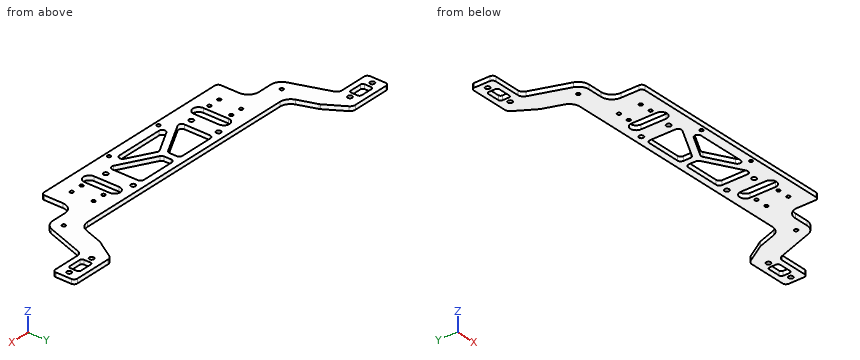
```python
from build123d import *

# Parameters (mm, degrees)
SKETCH_1_W           = 196
SKETCH_1_H           = 49.67
EXTRUDE_1_DEPTH      = 4
EXTRUDE_2_DEPTH      = 4
FILLET_1_R           = 10
FILLET_2_R           = 3
SKETCH_4_R           = 2.1
CUT_EXTRUDE_2_DEPTH  = 4
FILLET_3_R           = 5
SKETCH_5_R           = 1.55
CUT_EXTRUDE_3_DEPTH  = 10
SKETCH_7_R           = 2.05
CUT_EXTRUDE_5_DEPTH  = 102
CUT_EXTRUDE_8_DEPTH  = 10
FILLET_4_R           = 3
SKETCH_15_W          = 6
SKETCH_15_H          = 20
EXTRUDE_4_DEPTH      = 4
FILLET_11_R          = 10
FILLET_12_R          = 2
SKETCH_16_R          = 1.6
CUT_EXTRUDE_13_DEPTH = 10
SKETCH_23_W          = 16
SKETCH_23_H          = 22
CUT_EXTRUDE_17_DEPTH = 10
SKETCH_24_R          = 1.6
EXTRUDE_6_DEPTH      = 4
FILLET_14_R          = 10
SKETCH_25_W          = 15
SKETCH_25_H          = 10
CUT_EXTRUDE_18_DEPTH = 10
SKETCH_27_R          = 1.55
CUT_EXTRUDE_19_DEPTH = 5
SKETCH_30_R          = 1.6
CUT_EXTRUDE_22_DEPTH = 10
FILLET_15_R          = 2
CUT_EXTRUDE_23_DEPTH = 10


with BuildPart() as part:
    # 草图1 → 凸台-拉伸1 (new body)
    with BuildSketch(Plane.XY):
        Rectangle(SKETCH_1_W, SKETCH_1_H)
    extrude(amount=EXTRUDE_1_DEPTH)

    # 草图2 → 凸台-拉伸2 (add)
    with BuildSketch(Plane.XY.offset(4)):
        Polygon((98, 24.835), (114, 24.835), (122.222543405, 48.715), (134.566612912, 68.715), (174.566612912, 68.715), (174.566612912, 48.715), (143.374957029, 48.715), (128.265861358, 4.835), (98, 4.835), align=None)
        Polygon((-98, 24.835), (-98, 4.835), (-128.265861358, 4.835), (-143.374957029, 48.715), (-174.566612912, 48.715), (-174.566612912, 68.715), (-134.566612912, 68.715), (-122.222543405, 48.715), (-114, 24.835), align=None)
    extrude(amount=-EXTRUDE_2_DEPTH)

    # 圆角1
    fillet_1_edges = [part.edges().sort_by_distance(p)[0] for p in [
        (128.265861358, 4.835, 2),
        (114, 24.835, 2),
        (-128.265861358, 4.835, 2),
        (-114, 24.835, 2),
    ]]
    fillet(fillet_1_edges, radius=FILLET_1_R)

    # 圆角2
    fillet_2_edges = [part.edges().sort_by_distance(p)[0] for p in [
        (174.566612912, 48.715, 2),
        (174.566612912, 68.715, 2),
        (-174.566612912, 68.715, 2),
        (-174.566612912, 48.715, 2),
        (98, -24.835, 2),
        (-98, -24.835, 2),
    ]]
    fillet(fillet_2_edges, radius=FILLET_2_R)

    # 草图4 → 切除-拉伸2 (cut)
    with BuildSketch(Plane.XY.offset(4)):
        with Locations((47.5, -7.338706147)):
            Circle(SKETCH_4_R)
        with Locations((47.5, 17.661293853)):
            Circle(SKETCH_4_R)
        with Locations((-47.5, 17.661293853)):
            Circle(SKETCH_4_R)
        with Locations((-47.5, -7.338706147)):
            Circle(SKETCH_4_R)
    extrude(amount=-CUT_EXTRUDE_2_DEPTH, mode=Mode.SUBTRACT)

    # 圆角3
    fillet_3_edges = [part.edges().sort_by_distance(p)[0] for p in [
        (143.374957029, 48.715, 2),
        (134.566612912, 68.715, 2),
        (122.222543405, 48.715, 2),
        (-122.222543405, 48.715, 2),
        (-134.566612912, 68.715, 2),
        (-143.374957029, 48.715, 2),
    ]]
    fillet(fillet_3_edges, radius=FILLET_3_R)

    # 草图5 → 切除-拉伸3 (cut)
    with BuildSketch(Plane.XY.offset(4)):
        with Locations((27.5, -20.895)):
            Circle(SKETCH_5_R)
        with Locations(Location((-27.5, -20.895, 0), (0, 0, 180))):
            Circle(SKETCH_5_R)
    extrude(amount=-CUT_EXTRUDE_3_DEPTH, mode=Mode.SUBTRACT)

    # 草图7 → 切除-拉伸5 (cut)
    with BuildSketch(Plane.XY.offset(4)):
        with Locations((-168.566612912, 58.715)):
            Circle(SKETCH_7_R)
        with Locations((-143.566612912, 58.715)):
            Circle(SKETCH_7_R)
        with Locations(Location((143.566612912, 58.715, 0), (0, 0, 180))):
            Circle(SKETCH_7_R)
        with Locations(Location((168.566612912, 58.715, 0), (0, 0, 180))):
            Circle(SKETCH_7_R)
    extrude(amount=-CUT_EXTRUDE_5_DEPTH, mode=Mode.SUBTRACT)

    # 草图8 → 切除-拉伸8 (cut)
    with BuildSketch(Plane.XY.offset(4)):
        Polygon((-40, 18.835), (-40, -12.480899084), (-3, 7.619350916), (-3, 18.835), align=None)
        Polygon((0, 2.420899084), (-33.715414789, -15.895), (33.715414789, -15.895), align=None)
        Polygon((3, 7.619350916), (40, -12.480899084), (40, 18.835), (3, 18.835), align=None)
    extrude(amount=-CUT_EXTRUDE_8_DEPTH, mode=Mode.SUBTRACT)

    # 圆角4
    fillet_4_edges = [part.edges().sort_by_distance(p)[0] for p in [
        (0, 2.420899084, 2),
        (33.715414789, -15.895, 2),
        (-33.715414789, -15.895, 2),
        (3, 7.619350916, 2),
        (3, 18.835, 2),
        (40, 18.835, 2),
        (40, -12.480899084, 2),
        (-3, 7.619350916, 2),
        (-40, -12.480899084, 2),
        (-40, 18.835, 2),
        (-3, 18.835, 2),
    ]]
    fillet(fillet_4_edges, radius=FILLET_4_R)

    # 草图15 → 凸台-拉伸4 (add)
    with BuildSketch(Plane(origin=(0, 0, 0), x_dir=(-1, 0, 0), z_dir=(0, 0, -1))):
        with Locations((-101, -5.165)):
            Rectangle(SKETCH_15_W, SKETCH_15_H)
    extrude_4 = extrude(amount=-EXTRUDE_4_DEPTH)

    # 镜向5: 凸台-拉伸4 across plane
    add(extrude_4.mirror(Plane(origin=(0, 0, 0), x_dir=(0, 0, 1), z_dir=(1, 0, 0))))

    # 圆角11
    fillet_11_edges = [part.edges().sort_by_distance(p)[0] for p in [
        (104, 4.835, 2),
        (-104, 4.835, 2),
    ]]
    fillet(fillet_11_edges, radius=FILLET_11_R)

    # 圆角12
    fillet_12_edges = [part.edges().sort_by_distance(p)[0] for p in [
        (98, -15.165, 2),
        (104, -15.165, 2),
        (-104, -15.165, 2),
        (-98, -15.165, 2),
    ]]
    fillet(fillet_12_edges, radius=FILLET_12_R)

    # 草图16 → 切除-拉伸13 (cut)
    with BuildSketch(Plane.XY.offset(4)):
        with Locations((104, -10.165)):
            Circle(SKETCH_16_R)
        with Locations((104, 9.835)):
            Circle(SKETCH_16_R)
    cut_extrude_13 = extrude(amount=-CUT_EXTRUDE_13_DEPTH, mode=Mode.SUBTRACT)

    # 镜向6: 切除-拉伸13 across plane
    add(cut_extrude_13.mirror(Plane(origin=(0, 0, 0), x_dir=(0, 0, 1), z_dir=(1, 0, 0))), mode=Mode.SUBTRACT)

    # 草图23 → 切除-拉伸17 (cut)
    with BuildSketch(Plane.XY.offset(4)):
        with Locations((-106, -6.165)):
            Rectangle(SKETCH_23_W, SKETCH_23_H)
        with Locations((106, -6.165)):
            Rectangle(SKETCH_23_W, SKETCH_23_H)
    extrude(amount=-CUT_EXTRUDE_17_DEPTH, mode=Mode.SUBTRACT)

    # 草图24 → 凸台-拉伸6 (add)
    with BuildSketch(Plane.XY.offset(4)):
        with Locations((104, 9.835)):
            Circle(SKETCH_24_R)
        with Locations((-104, 9.835)):
            Circle(SKETCH_24_R)
    extrude(amount=-EXTRUDE_6_DEPTH)

    # 圆角14
    fillet_14_edges = [part.edges().sort_by_distance(p)[0] for p in [
        (-98, 4.835, 2),
        (98, 4.835, 2),
    ]]
    fillet(fillet_14_edges, radius=FILLET_14_R)

    # 草图25 → 切除-拉伸18 (cut)
    with BuildSketch(Plane.XY.offset(4)):
        with Locations((-156.066612912, 58.715)):
            Rectangle(SKETCH_25_W, SKETCH_25_H)
        with Locations((156.066612912, 58.715)):
            Rectangle(SKETCH_25_W, SKETCH_25_H)
    extrude(amount=-CUT_EXTRUDE_18_DEPTH, mode=Mode.SUBTRACT)

    # 草图27 → 切除-拉伸19 (cut)
    with BuildSketch(Plane(origin=(0, 0, 0), x_dir=(-1, 0, 0), z_dir=(0, 0, -1))):
        with Locations((-82, -10.165)):
            Circle(SKETCH_27_R)
        with Locations((-82, 9.835)):
            Circle(SKETCH_27_R)
        with Locations((82, 9.835)):
            Circle(SKETCH_27_R)
        with Locations((82, -10.165)):
            Circle(SKETCH_27_R)
        with Locations((-71, 9.835)):
            Circle(SKETCH_27_R)
        with Locations((-71, -10.165)):
            Circle(SKETCH_27_R)
        with Locations((71, -10.165)):
            Circle(SKETCH_27_R)
        with Locations((71, 9.835)):
            Circle(SKETCH_27_R)
    extrude(amount=-CUT_EXTRUDE_19_DEPTH, mode=Mode.SUBTRACT)

    # 草图30 → 切除-拉伸22 (cut)
    with BuildSketch(Plane.XY.offset(4)):
        with Locations((121.132930679, 14.835)):
            Circle(SKETCH_30_R)
        with Locations(Location((-121.132930679, 14.835, 0), (0, 0, 180))):
            Circle(SKETCH_30_R)
    extrude(amount=-CUT_EXTRUDE_22_DEPTH, mode=Mode.SUBTRACT)

    # 圆角15
    fillet_15_edges = [part.edges().sort_by_distance(p)[0] for p in [
        (-148.566612912, 63.715, 2),
        (-148.566612912, 53.715, 2),
        (-163.566612912, 53.715, 2),
        (-163.566612912, 63.715, 2),
        (163.566612912, 63.715, 2),
        (163.566612912, 53.715, 2),
        (148.566612912, 53.715, 2),
        (148.566612912, 63.715, 2),
    ]]
    fillet(fillet_15_edges, radius=FILLET_15_R)

    # 草图31 → 切除-拉伸23 (cut)
    with BuildSketch(Plane.XY.offset(4)):
        with BuildLine():
            Line((66, 11.5), (66, -11.5))
            ThreePointArc((66, -11.5), (60.75, -16.75), (55.5, -11.5))
            Line((55.5, -11.5), (55.5, 11.5))
            ThreePointArc((55.5, 11.5), (60.75, 16.75), (66, 11.5))
        make_face()
        with BuildLine():
            Line((-66, 11.5), (-66, -11.5))
            ThreePointArc((-66, -11.5), (-60.75, -16.75), (-55.5, -11.5))
            Line((-55.5, -11.5), (-55.5, 11.5))
            ThreePointArc((-55.5, 11.5), (-60.75, 16.75), (-66, 11.5))
        make_face()
    extrude(amount=-CUT_EXTRUDE_23_DEPTH, mode=Mode.SUBTRACT)


solid = part.part
```
Check sheet for the modelled part. Datum: model origin and axes. Units: mm. Round coordinates to 2 decimals unless told otherwise and drop trailing zeros. Write each loop counter-clockwise with the first axis right and the second up, starting at its lowest first coordinate (ties: lowest second). Pieces come first, ordered by that corner, then holes. Notation, with made-up numbers: M 6.5,48.5 L 51.5,48.5 A13 cw 51.5,70.5 Z; hole C -34.5,43 d3. An arc over 180 degrees is marked long. Write item = value, one per line. Start each with the question number.
1. Section check C-C, the plane x = 113. Record the cut outline in (y, z) (3 decimals).
2. Gauge pin test, flat ends, axial feed: pin 1 (2.5 mm diameter, centred on x = -27.5, y = -20.895, fed in from +Z); pin 2 (1.2 mm diameter, centred on x = 153.5, z = 2.5, fed in from -Y) (3 decimals); pin 3 (1.2 mm diameter, centred on y = -1, z = 1.5, fed in from +X); pin 4 (2 mm diameter, centred on y = 0, z = 2, fed in from +X). Record the tip position at first contact, or that the pin passes through.
3. Section check A-A, the plane x = -60.75. Record the cut outline in (y, z) (3 decimals).
4. Section check B-B, the plane z = 2.45. State how many separate pieces and enclosed holes the cut face has, then the cut area to 3 significant figures.
5. Scan lines: line 1 (Y direction, x = -82, z = 1.6) (3 decimals); line 2 (X direction, y = -20.5, z = 0.5); line 3 (Y direction, x = 47, z = 1.1) (3 decimals). Record each from-to range of solid material in increasing order. Write a range as [from, to].
Results found:
q1.outline = M 4.835,0 L 26.936,0 L 26.936,4 L 4.835,4 Z
q2.pin_1 = through
q2.pin_2 = 48.715
q2.pin_3 = 99.21
q2.pin_4 = 100.13
q3.outline = M -24.835,0 L -16.75,0 L -16.75,4 L -24.835,4 Z; M 16.75,0 L 24.835,0 L 24.835,4 L 16.75,4 Z
q4.separate_pieces = 1
q4.enclosed_holes = 27
q4.area = 10,700 mm^2
q5.line_1 = [-24.835, -11.715], [-8.615, 8.285], [11.385, 24.835]
q5.line_2 = [-98, -29], [-26, 26], [29, 98]
q5.line_3 = [-24.835, -9.378], [-5.299, 15.622], [19.701, 24.835]
